Source: CAD feature listing. Evaluate the final solid. Frame: model axes, mm. Coordinates: 2 decimals unless noted, no trailing zeros. One line per question, with ' | ' between items. Start each with the question number.
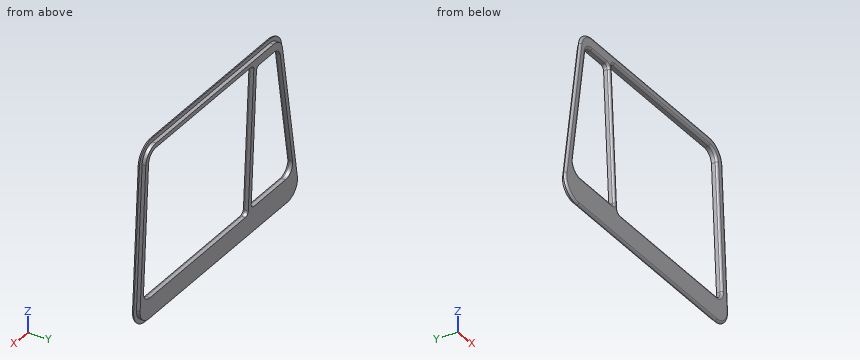
```python
from build123d import *

# Parameters (mm, degrees)
BOX024_W               = 11
BOX024_H               = 7
BOX024_DEPTH           = 48
BOX024_ROLL_ANGLE      = -2.200006
BOX024_PITCH_ANGLE     = 12.000025
BOX024_PLACEMENT_ANGLE = -1e-06
BOX023_W               = 17
BOX023_H               = 5
BOX023_DEPTH           = 34
BOX023_ROLL_ANGLE      = -2.2
FILLET024_R            = 2.5
FILLET025_R            = 1
BOX025_W               = 38
BOX025_H               = 5
BOX025_DEPTH           = 36
BOX025_ROLL_ANGLE      = -2.2
FILLET022_R            = 2.5
FILLET023_R            = 1
BOX003_W               = 11
BOX003_H               = 7
BOX003_DEPTH           = 48
BOX003_ROLL_ANGLE      = -2.200006
BOX003_PITCH_ANGLE     = 12.000025
BOX003_PLACEMENT_ANGLE = -1e-06
BOX002_W               = 58
BOX002_H               = 1
BOX002_DEPTH           = 42
BOX002_ROLL_ANGLE      = -2.2
FILLET021_R            = 3.5
BOX022_W               = 11
BOX022_H               = 7
BOX022_DEPTH           = 48
BOX022_ROLL_ANGLE      = -2.200006
BOX022_PITCH_ANGLE     = 12.000025
BOX022_PLACEMENT_ANGLE = -1e-06
BOX021_W               = 60
BOX021_H               = 0.5
BOX021_DEPTH           = 44
BOX021_ROLL_ANGLE      = -2.2
FILLET020_R            = 4.5
FILLET026_R            = 0.49
FILLET027_R            = 0.49


with BuildPart() as cube450:
    # Box024 → Box024 (new body)
    with BuildSketch(Plane.XY):
        with Locations((5.5, 3.5)):
            Rectangle(BOX024_W, BOX024_H)
    extrude(amount=BOX024_DEPTH)


with BuildPart() as cube450_1:
    # Box024 roll: moved
    add(cube450.part.rotate(Axis((0, 0, 0), (1, 0, 0)), BOX024_ROLL_ANGLE))


with BuildPart() as cube450_2:
    # Box024 pitch: moved
    add(cube450_1.part.rotate(Axis((0, 0, 0), (0, 1, 0)), BOX024_PITCH_ANGLE))


with BuildPart() as cube450_3:
    # Box024 placement: moved
    add(cube450_2.part.moved(Location((9.5, 1, 70))).rotate(Axis((9.5, 1, 70), (0, 0, 1)), BOX024_PLACEMENT_ANGLE))


with BuildPart() as fillet025:
    # Box023 → Box023 (new body)
    with BuildSketch(Plane.XY):
        with Locations((8.5, 2.5)):
            Rectangle(BOX023_W, BOX023_H)
    extrude(amount=BOX023_DEPTH)


with BuildPart() as fillet025_1:
    # Box023 roll: moved
    add(fillet025.part.rotate(Axis((0, 0, 0), (1, 0, 0)), BOX023_ROLL_ANGLE))


with BuildPart() as fillet025_2:
    # Box023 placement: moved
    add(fillet025_1.part.moved(Location((20.5, 2, 76))))

    # Cut016: cut Cube450
    add(cube450_3.part, mode=Mode.SUBTRACT)

    # Fillet024
    fillet024_edges = [fillet025_2.edges().sort_by_distance(p)[0] for p in [
        (22.000691, 4.498157, 75.90403),
        (29.222302, 5.803343, 109.87897),
    ]]
    fillet(fillet024_edges, radius=FILLET024_R)

    # Fillet025
    fillet025_edges = [fillet025_2.edges().sort_by_distance(p)[0] for p in [
        (37.5, 4.498157, 75.90403),
        (37.5, 5.803343, 109.87897),
    ]]
    fillet(fillet025_edges, radius=FILLET025_R)


with BuildPart() as fusion002:
    # Box025 → Box025 (new body)
    with BuildSketch(Plane.XY):
        with Locations((19, 2.5)):
            Rectangle(BOX025_W, BOX025_H)
    extrude(amount=BOX025_DEPTH)


with BuildPart() as fusion002_1:
    # Box025 roll: moved
    add(fusion002.part.rotate(Axis((0, 0, 0), (1, 0, 0)), BOX025_ROLL_ANGLE))


with BuildPart() as fusion002_2:
    # Box025 placement: moved
    add(fusion002_1.part.moved(Location((38.5, 2, 75))))

    # Fillet022
    fillet022_edges = [fusion002_2.edges().sort_by_distance(p)[0] for p in [
        (76.5, 5.880118, 110.877495),
        (76.5, 4.498157, 74.90403),
    ]]
    fillet(fillet022_edges, radius=FILLET022_R)

    # Fillet023
    fillet023_edges = [fusion002_2.edges().sort_by_distance(p)[0] for p in [
        (38.5, 4.498157, 74.90403),
        (38.5, 5.880118, 110.877495),
    ]]
    fillet(fillet023_edges, radius=FILLET023_R)

    # Fusion002: union Fillet025
    add(fillet025_2.part)


with BuildPart() as cube049:
    # Box003 → Box003 (new body)
    with BuildSketch(Plane.XY):
        with Locations((5.5, 3.5)):
            Rectangle(BOX003_W, BOX003_H)
    extrude(amount=BOX003_DEPTH)


with BuildPart() as cube049_1:
    # Box003 roll: moved
    add(cube049.part.rotate(Axis((0, 0, 0), (1, 0, 0)), BOX003_ROLL_ANGLE))


with BuildPart() as cube049_2:
    # Box003 pitch: moved
    add(cube049_1.part.rotate(Axis((0, 0, 0), (0, 1, 0)), BOX003_PITCH_ANGLE))


with BuildPart() as cube049_3:
    # Box003 placement: moved
    add(cube049_2.part.moved(Location((8.5, 1, 70))).rotate(Axis((8.5, 1, 70), (0, 0, 1)), BOX003_PLACEMENT_ANGLE))


with BuildPart() as fillet021:
    # Box002 → Box002 (new body)
    with BuildSketch(Plane.XY):
        with Locations((29, 0.5)):
            Rectangle(BOX002_W, BOX002_H)
    extrude(amount=BOX002_DEPTH)


with BuildPart() as fillet021_1:
    # Box002 roll: moved
    add(fillet021.part.rotate(Axis((0, 0, 0), (1, 0, 0)), BOX002_ROLL_ANGLE))


with BuildPart() as fillet021_2:
    # Box002 placement: moved
    add(fillet021_1.part.moved(Location((19.5, 3, 70))))

    # Cut001: cut Cube049
    add(cube049_3.part, mode=Mode.SUBTRACT)

    # Fillet021
    fillet021_edges = [fillet021_2.edges().sort_by_distance(p)[0] for p in [
        (77.5, 3.499631, 69.980806),
        (19.741668, 3.499631, 69.980806),
        (77.5, 5.111919, 111.949849),
        (28.662482, 5.111919, 111.949849),
    ]]
    fillet(fillet021_edges, radius=FILLET021_R)


with BuildPart() as cube448:
    # Box022 → Box022 (new body)
    with BuildSketch(Plane.XY):
        with Locations((5.5, 3.5)):
            Rectangle(BOX022_W, BOX022_H)
    extrude(amount=BOX022_DEPTH)


with BuildPart() as cube448_1:
    # Box022 roll: moved
    add(cube448.part.rotate(Axis((0, 0, 0), (1, 0, 0)), BOX022_ROLL_ANGLE))


with BuildPart() as cube448_2:
    # Box022 pitch: moved
    add(cube448_1.part.rotate(Axis((0, 0, 0), (0, 1, 0)), BOX022_PITCH_ANGLE))


with BuildPart() as cube448_3:
    # Box022 placement: moved
    add(cube448_2.part.moved(Location((7.5, 1, 70))).rotate(Axis((7.5, 1, 70), (0, 0, 1)), BOX022_PLACEMENT_ANGLE))


with BuildPart() as left_front_window_border:
    # Box021 → Box021 (new body)
    with BuildSketch(Plane.XY):
        with Locations((30, 0.25)):
            Rectangle(BOX021_W, BOX021_H)
    extrude(amount=BOX021_DEPTH)


with BuildPart() as left_front_window_border_1:
    # Box021 roll: moved
    add(left_front_window_border.part.rotate(Axis((0, 0, 0), (1, 0, 0)), BOX021_ROLL_ANGLE))


with BuildPart() as left_front_window_border_2:
    # Box021 placement: moved
    add(left_front_window_border_1.part.moved(Location((18.5, 2.6, 69))))

    # Cut015: cut Cube448
    add(cube448_3.part, mode=Mode.SUBTRACT)

    # Fillet020
    fillet020_edges = [left_front_window_border_2.edges().sort_by_distance(p)[0] for p in [
        (78.5, 2.849816, 68.990403),
        (18.531151, 2.849816, 68.990403),
        (78.5, 4.538879, 112.957971),
        (27.876766, 4.538879, 112.957971),
    ]]
    fillet(fillet020_edges, radius=FILLET020_R)

    # Fusion: union Fillet021
    add(fillet021_2.part)

    # Cut017: cut Fusion002
    add(fusion002_2.part, mode=Mode.SUBTRACT)

    # Fillet026
    fillet026_edges = [left_front_window_border_2.edges().sort_by_distance(p)[0] for p in [
        (33.880234, 4.172818, 109.941608),
        (56.75, 4.211234, 110.941608),
    ]]
    fillet(fillet026_edges, radius=FILLET026_R)

    # Fillet027
    fillet027_edges = [left_front_window_border_2.edges().sort_by_distance(p)[0] for p in [
        (49.044763, 2.6, 69),
    ]]
    fillet(fillet027_edges, radius=FILLET027_R)


solid = left_front_window_border_2.part
```
(1) Ray query, L1, parallel to X at y = 5.1, z = 104; L2, parallel to X at y = 5, z = 102; L3, parallel to Y at x = 28, z = 109. Return the intervals inside material, ascending.
(2) Contact query for flat-ended pins moving along their axis: pin 1 Ø12 at (x, z) = (60.5, 75.5) entering from +Y; pin 2 Ø10 at (x, z) = (36.5, 75.5) entering from -Y; pin 3 Ø1.5 at (y, z) = (4.5, 83.5) entering from -X; pin 4 Ø1.7 at (y, z) = (4, 91.5) entering from +X. Output: stop coordinate, or through.
(3) Cut plane B-B, the plane z = 85. State how many separate pieces and enclosed holes the cut face has, and give its area (3 significant figures).
Here are the results:
1) L1: x = 26.97 to 27.97, 37.5 to 38.5, 76.5 to 77.5 | L2: x = 26.55 to 27.55, 37.5 to 38.5, 76.5 to 77.5 | L3: y = 4.14 to 4.64
2) pin 1: stops at y = 4.19 | pin 2: stops at y = 2.66 | pin 3: stops at x = 22.46 | pin 4: stops at x = 78.5
3) separate pieces: 3 | enclosed holes: 0 | area: 4.78 mm2
